Design review of the part built by this model. Coordinates are the model's own, in mm. Coordinates: 2 decimals unless noted, no trailing zeros. Loops run counter-clockwise (first coordinate to the right, second up) from the corner with the lowest first, then second, coordinate; pieces in that order, holes last. Notation, with made-up numbers: (-29, -36.75) -> (0, -36.75) arc R22 cw to (0, -30.75) -> close; hole circle Ø9 at (-29, 71). An arc over 180 degrees is marked (long way). One line per item, written item: value. Start each with the question number.
1. For probe 1 along Y at (x, z) = (0, 3.25); probe 2 along Z at (x, y) = (-0.35, 1.55); probe 3 along X at (y, z) = (1.35, 5.5), list the stretches that pass through material, from the lowest coordinate up.
2. Add section B-B on z = 8.5. Write out the cut boundary in (x, y).
3. Add section A-A on x = 0. Write out the cut boundary in (y, z), plus the area to 4 significant figures.
4. Add section C-C on y = -1.8. Write out the cut boundary in (x, z), plus the area to 3 significant figures.
```python
from build123d import *

# Parameters (mm, degrees)
F0_R     = 2.5
F1_DEPTH = 14.25
F3_D     = 4
F3_DEPTH = 2
F3_TIP   = 1.2017212381
F4_R     = 2.1505871319
F5_DEPTH = 4.5


with BuildPart() as f1:
    # F0 (on Top) → F1 (new body)
    with BuildSketch(Plane.XY):
        Circle(F0_R)
        with BuildLine():
            ThreePointArc((-1.5, 1.3228756555), (2, 0), (-1.5, -1.3228756555))
            Line((-1.5, -1.3228756555), (-1.5, 1.3228756555))
        make_face(mode=Mode.SUBTRACT)
    extrude(amount=F1_DEPTH)

    # F3
    with Locations(Plane(origin=(0, 0, 0), x_dir=(1, 0, 0), z_dir=(0, 0, -1))):
        with Locations((0, 0)):
            Hole(F3_D / 2, depth=F3_DEPTH)
            with Locations((0, 0, -(F3_DEPTH + F3_TIP / 2))):  # 118° drill point
                Cone(0, F3_D / 2, F3_TIP, mode=Mode.SUBTRACT)

    # F4 (on face) → F5 (join)
    with BuildSketch(Plane.XY.offset(14.25)):
        Circle(F4_R)
        with BuildLine():
            Line((-1.5, -1.3228756555), (-1.5, 1.3228756555))
            ThreePointArc((-1.5, 1.3228756555), (2, 0), (-1.5, -1.3228756555))
        make_face(mode=Mode.SUBTRACT)
        with BuildLine():
            ThreePointArc((-1.5, -1.3228756555), (2, 0), (-1.5, 1.3228756555))
            Line((-1.5, 1.3228756555), (-1.5, -1.3228756555))
        make_face()
    extrude(amount=-F5_DEPTH)


solid = f1.part
```
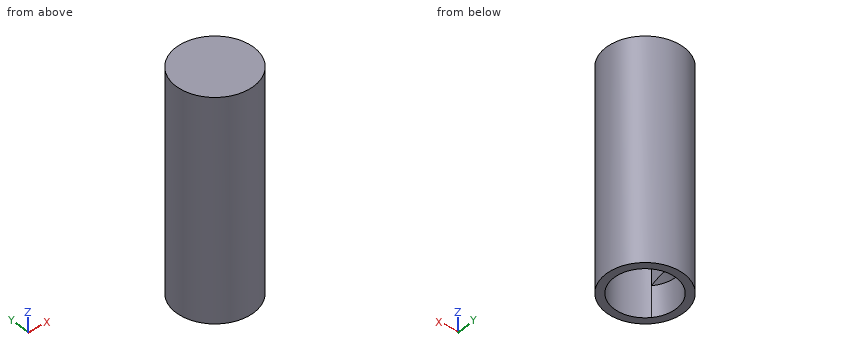
Worked answers:
1. probe 1: y = -2.5 to -2, 2 to 2.5
1. probe 2: z = 9.75 to 14.25
1. probe 3: x = -2.1 to -1.48, 1.48 to 2.1
2. outline: circle Ø5 at (0, 0); hole (-1.5, -1.32) arc R2 ccw (long way) to (-1.5, 1.32) -> close
3. outline: (-2.5, 0) -> (-2, 0) -> (-2, 9.75) -> (2, 9.75) -> (2, 0) -> (2.5, 0) -> (2.5, 14.25) -> (-2.5, 14.25) -> close
3. area: 32.25 mm²
4. outline: (-1.73, 0) -> (-0.87, 0) -> (-0.87, 9.75) -> (0.87, 9.75) -> (0.87, 0) -> (1.73, 0) -> (1.73, 14.25) -> (-1.73, 14.25) -> close
4. area: 32.4 mm²
